```python
from build123d import *

# Parameters (mm, degrees)
SKETCH2_R                = 14.478
BOSS_EXTRUDE1_DEPTH      = 50.8
CUT_EXTRUDE3_DEPTH       = 38.1
BOSS_EXTRUDE2_DEPTH      = 12.7
BOSS_EXTRUDE2_DEPTH_BACK = 12.7
SKETCH16_R               = 14.478
CUT_EXTRUDE4_START       = -19.05
CUT_EXTRUDE4_DEPTH       = 19.05


# Read off the part's stored shape, not the designer's step: Cut-Extrude4
with BuildPart() as part:
    # Sketch2 → Boss-Extrude1 (new body)
    with BuildSketch(Plane(origin=(0, 0, 0), x_dir=(1, 0, 0), z_dir=(0, 1, 0))):
        with Locations(Location((0, 0, 0), (0, 0, 270))):
            Circle(SKETCH2_R)
        with BuildLine():
            Line((-13.081, 3.175), (-8.059107313, -1.349826056))
            ThreePointArc((-8.059107313, -1.349826056), (0, -4.445), (8.059107313, -1.349826056))
            Line((8.059107313, -1.349826056), (13.081, 3.175))
            ThreePointArc((13.081, 3.175), (13.146371637, 4.430535164), (11.890836473, 4.495906802))
            Line((11.890836473, 4.495906802), (6.868943786, -0.028919255))
            ThreePointArc((6.868943786, -0.028919255), (0, -2.667), (-6.868943786, -0.028919255))
            Line((-6.868943786, -0.028919255), (-11.890836473, 4.495906802))
            ThreePointArc((-11.890836473, 4.495906802), (-13.146371637, 4.430535164), (-13.081, 3.175))
        make_face(mode=Mode.SUBTRACT)
    extrude(amount=BOSS_EXTRUDE1_DEPTH)

    # Sketch15 → Cut-Extrude3 (cut)
    with BuildSketch(Plane.XZ):
        with BuildLine():
            ThreePointArc((13.081, -3.175), (13.146371637, -4.430535164), (11.890836473, -4.495906802))
            Line((11.890836473, -4.495906802), (13.285944291, -5.752926933))
            ThreePointArc((13.285944291, -5.752926933), (14.176854119, -2.937565536), (14.478, 0))
            ThreePointArc((14.478, 0), (-2.937565536, 14.176854119), (-13.285944291, -5.752926933))
            Line((-13.285944291, -5.752926933), (-11.890836473, -4.495906802))
            ThreePointArc((-11.890836473, -4.495906802), (-13.146371637, -4.430535164), (-13.081, -3.175))
            Line((-13.081, -3.175), (-8.059107313, 1.349826056))
            ThreePointArc((-8.059107313, 1.349826056), (0, 4.445), (8.059107313, 1.349826056))
            Line((8.059107313, 1.349826056), (13.081, -3.175))
        make_face()
    extrude(amount=-CUT_EXTRUDE3_DEPTH, mode=Mode.SUBTRACT)

    # Sketch16 → Boss-Extrude2 (add, two sides: drawn at the far end of the back side and taken through both)
    with BuildSketch(Plane(origin=(0, 50.8, 0), x_dir=(1, 0, 0), z_dir=(0, 1, 0)).offset(-BOSS_EXTRUDE2_DEPTH_BACK)):
        with Locations(Location((0, 0, 0), (0, 0, 156.586977838))):
            Circle(SKETCH16_R)
    extrude(amount=BOSS_EXTRUDE2_DEPTH + BOSS_EXTRUDE2_DEPTH_BACK)

    # Cut-Extrude4 outline → Cut-Extrude4 (cut)
    with BuildSketch(Plane(origin=(0, 63.5, 0), x_dir=(1, 0, 0), z_dir=(0, 1, 0)).offset(CUT_EXTRUDE4_START)):
        with BuildLine():
            ThreePointArc((-9.525, -10.903525072), (0, -14.478), (9.525, -10.903525072))
            Line((9.525, -10.903525072), (9.525, 4.572))
            Line((9.525, 4.572), (-9.525, 4.572))
            Line((-9.525, 4.572), (-9.525, -10.903525072))
        make_face()
    extrude(amount=CUT_EXTRUDE4_DEPTH, mode=Mode.SUBTRACT)


solid = part.part
```
Verification items for the finished model (mm, model axes). A direction names the side the tool comes from. Coordinates: 2 decimals unless noted, no trailing zeros. Write each loop counter-clockwise with the first axis right and the second up, starting at its lowest first coordinate (ties: lowest second). Pieces come first, ordered by that corner, then holes. Notation, with made-up numbers: (-15, 36.25) - (9, 36.25) arc R28 cw to (9, 62.25) - close; hole circle Ø10 at (40.25, -28.75). An arc over 180 degrees is marked (long way). One line per question, with ' | ' between items. Start each with the question number.
1. Access from +Z, -Z, +X, -X, +Y, -Y to the whole of each face (thin tool, end or side, straight path). Record for faces 4 (the flat face through (0, 63.5, -7)), 5 (the flat face through (0, 54, -4.572)).
2. Section check B-B (x = 0). Enter the section's corners in (y, z).
3. Gauge pin test, flat ends, axial feed: P1, Ø8, axis at x = 7.5, z = -3.5, coming from the +Y side; P2, Ø1, axis at x = 8, z = -2.5, coming from the +Y side; P3, Ø6, axis at y = 30.5, z = 4, coming from the -X side; P4, Ø4, axis at y = 50.5, z = 6.5, coming from the +X side. Record the tip position at first contact, or that the pin passes through.
4. Draft check along X on faces 1 (the flat face through (0, 44.45, 5)), 2 (the cylindrical face through (0.105, 18.783, 2.666)), 3 (the flat face through (0, 38.1, 5)). Enter one of: released by +X, released by -X, zero draft, split by the parting line, or undercut.
5. Material ranges on line 1 along X through (y, z) = (55, -4.25) (3 decimals); line 2 along X through (y, z) = (51, 6.75) (3 decimals); line 3 along Y through (x, z) = (3.5, 0.75), recorded low to high.
6. Section check A-A (y = 27). Enter the section's corners in (x, z).
7. Section check C-C (z = -10.25). Enter the section's corners in (x, y).
8. Section check D-D (x = 7.5). Enter the section's corners in (y, z).
Computed values:
1) face 4: +Z, -Z, +X, -X, +Y | face 5: +Z, +Y
2) outline: (0, -14.48) - (63.5, -14.48) - (63.5, -4.57) - (44.45, -4.57) - (44.45, 14.48) - (38.1, 14.48) - (38.1, 2.67) - (0, 2.67) - close
3) P1: y = 63.5 | P2: y = 44.45 | P3: x = -5.61 | P4: x = 13.76
4) face 1: undercut | face 2: split by the parting line | face 3: zero draft
5) line 1: -13.84 to -9.525, 9.525 to 13.84 | line 2: -12.808 to -9.525, 9.525 to 12.808 | line 3: 0 to 44.45
6) outline: (-13.29, -5.75) arc R14.48 ccw to (13.29, -5.75) - (6.87, 0.03) arc R10.26 ccw to (-6.87, 0.03) - close
7) outline: (-10.22, 0) - (10.22, 0) - (10.22, 63.5) - (-10.22, 63.5) - close
8) outline: (0, -12.38) - (63.5, -12.38) - (63.5, -4.57) - (44.45, -4.57) - (44.45, 12.38) - (38.1, 12.38) - (38.1, -0.54) - (0, -0.54) - close
